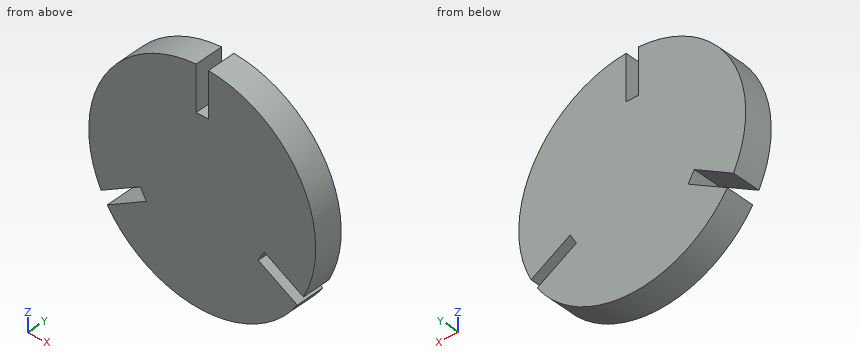
from build123d import *

# Parameters (mm, degrees)
F1_DEPTH = 6.35


with BuildPart() as f1:
    # F0 (on Front) → F1 (new body)
    with BuildSketch(Plane.XZ):
        with BuildLine():
            Line((-1.35, 15), (-1.35, 24.963523))
            ThreePointArc((-1.35, 24.963523), (-21.650635, 12.5), (-22.294045, -11.312627))
            Line((-22.294045, -11.312627), (-13.665381, -6.330866))
            Line((-13.665381, -6.330866), (-12.315381, -8.669134))
            Line((-12.315381, -8.669134), (-20.944045, -13.650896))
            ThreePointArc((-20.944045, -13.650896), (0, -25), (20.944045, -13.650896))
            Line((20.944045, -13.650896), (12.315381, -8.669134))
            Line((12.315381, -8.669134), (13.665381, -6.330866))
            Line((13.665381, -6.330866), (22.294045, -11.312627))
            ThreePointArc((22.294045, -11.312627), (21.650635, 12.5), (1.35, 24.963523))
            Line((1.35, 24.963523), (1.35, 15))
            Line((1.35, 15), (-1.35, 15))
        make_face()
    extrude(amount=F1_DEPTH)


solid = f1.part
Can you work these out from the model? Positions are in its coordinate system, mm. Give positions to 0.01 mm unless a question says otherwise; leave off trailing zeros. Loops run counter-clockwise (first coordinate to the right, second up) from the corner with the lowest first, then second, coordinate; pieces in that order, holes last. Notation, with made-up numbers: M 12.5,-1.75 L 53.5,-1.75 A19 cw 53.5,19.25 Z; hole C -7.75,-28.75 d2. An arc over 180 degrees is marked long. One line per item, written item: value. Start each with the question number.
1) If I drill on line 1 (Z direction, x = -15.5, y = -2); line 2 (Z direction, x = -20, y = -1.5); line 3 (X direction, y = -2.5, z = -0.5) (3 decimals), over which ranges is the centre line in solid material (lowest first)? Write a range as [from, to].
2) I'm going to push flat-ended pins straight in: pin 1 (3 mm diameter, centred on y = -3.5, z = 22, fed in from +X); pin 2 (1 mm diameter, centred on x = 14.5, y = -4, fed in from -Z); pin 3 (3 mm diameter, centred on x = -13.5, z = 0.5, fed in from +Y); pin 4 (3 mm diameter, centred on y = -1.5, z = 8, fed in from +X). Where does each tip first touch, or does it pass through?
3) If we section it at B-B, the plane z = -7.5: Write out the boundary of the cut face in (x, y).
4) If we section it at C-C, the plane x = -19: Write out the boundary of the cut face in (y, z).
5) If we section it at D-D, the plane x = -7: Write out the boundary of the cut face in (y, z).
6) If we section it at A-A, the plane y = -2.75: Write out the boundary of the cut face in (x, z).
Completed:
1. line 1: z = [-19.62, -10.51], [-7.39, 19.62]
1. line 2: z = [-15, -13.11], [-9.99, 15]
1. line 3: x = [-24.995, 24.995]
2. pin 1: stops at x = 14.31
2. pin 2: stops at z = -20.71
2. pin 3: stops at y = 0
2. pin 4: stops at x = 24.14
3. outline: M -23.85,-6.35 L -15.69,-6.35 L -15.69,0 L -23.85,0 Z; M -12.99,-6.35 L 12.99,-6.35 L 12.99,0 L -12.99,0 Z; M 15.69,-6.35 L 23.85,-6.35 L 23.85,0 L 15.69,0 Z
4. outline: M -6.35,-16.25 L 0,-16.25 L 0,-12.53 L -6.35,-12.53 Z; M -6.35,-9.41 L 0,-9.41 L 0,16.25 L -6.35,16.25 Z
5. outline: M -6.35,-24 L 0,-24 L 0,24 L -6.35,24 Z
6. outline: M -22.29,-11.31 L -13.67,-6.33 L -12.32,-8.67 L -20.94,-13.65 A25 ccw 20.94,-13.65 L 12.32,-8.67 L 13.67,-6.33 L 22.29,-11.31 A25 ccw 1.35,24.96 L 1.35,15 L -1.35,15 L -1.35,24.96 A25 ccw Z
